Build history of the part. All positions in model axes, mm. A direction names the side the tool comes from. Give positions to 0.01 mm unless a question says otherwise; leave off trailing zeros. Order: outer loops, then holes, each group sorted by start corner. A loop starts at its lowest first (then second) coordinate and runs counter-clockwise, first axis right, second up. Notation, with made-up numbers: M 49,-18 L 77,-18 A21 cw 77,17 Z; hole C 82.5,-4.75 d8. An arc over 180 degrees is marked long. Answer as CSV lines item,"result".
from build123d import *

# Parameters (mm, degrees)
F0_R      = 185
F1_DEPTH  = 25
F2_R      = 100
F2_R_2    = 65
F3_DEPTH  = 30
F3_FACE_R = 65
F4_DEPTH  = 25.001


with BuildPart() as f1:
    # F0 (on Top) → F1 (new body)
    with BuildSketch(Plane.XY):
        Circle(F0_R)
    extrude(amount=F1_DEPTH)

    # F2 (on face) → F3 (join)
    with BuildSketch(Plane.XY.offset(25)):
        Circle(F2_R)
        Circle(F2_R_2, mode=Mode.SUBTRACT)
    extrude(amount=F3_DEPTH)

    # F3_face (on face) → F4 (cut, through all)
    with BuildSketch(Plane.XY.offset(25)):
        Circle(F3_FACE_R)
    extrude(amount=-F4_DEPTH, mode=Mode.SUBTRACT)


solid = f1.part
Item 1: 3-axis set-ups, long thin cutter, end or side, ignore diameter. For faces 1 (the cylindrical face through (95.38, 30.04, 39.79)), 2 (the cylindrical face through (99.455, 155.993, 12.325)): which of +Z, -Z, +X, -X, +Y, -Y reach the whole face in a straight line?
Geometry says:
face 1,"+Z"
face 2,"+Z, -Z"
Item 2: Drop flat-ended pins along their axis: pin 1 (2 mm diameter, centred on x = -112, z = 7.5, fed in from -Y); pin 2 (6 mm diameter, centred on x = -120.5, y = -124.5, fed in from +Z); pin 3 (2 mm diameter, centred on x = -60, z = 20, fed in from +Y). Give the stop position or say it passes through.
Geometry says:
pin 1,"stops at y = -148"
pin 2,"stops at z = 25"
pin 3,"stops at y = 175.34"
Item 3: Band-saw the part on C-C (z = 49). Give the cut face in (x, y), and give its area (3 significant figures).
Geometry says:
outline,"C 0,0 d200; hole C 0,0 d130"
area,"18,100 mm2"
Item 4: Probe line 1 along Y through (x, z) = (0, 38.25); line 2 along Z through (x, y) = (95.5, 58.5); line 3 along Y through (x, z) = (0, 11). List the from-to ranges inside material, lowest first. Write a range as from..to.
Geometry says:
line 1,"y = -100..-65, 65..100"
line 2,"z = 0..25"
line 3,"y = -185..-65, 65..185"
Item 5: Band-saw the part on D-D (y = 88). Give the cut face in (x, z), and give its area (3 significant figures).
Geometry says:
outline,"M -162.73,0 L 162.73,0 L 162.73,25 L 47.5,25 L 47.5,55 L -47.5,55 L -47.5,25 L -162.73,25 Z"
area,"11,000 mm2"
Item 6: Band-saw the part on A-A (x = 0). Give the cut face in (y, z), and give its area (3 significant figures).
Geometry says:
outline,"M -185,0 L -65,0 L -65,55 L -100,55 L -100,25 L -185,25 Z; M 65,0 L 185,0 L 185,25 L 100,25 L 100,55 L 65,55 Z"
area,"8,100 mm2"
